```python
from build123d import *

# Parameters (mm, degrees)
ESQUISSE1_R                  = 70
BOSS_EXTRU_1_DEPTH           = 10
CHANFREIN1_SIZE              = 2.12
CHANFREIN1_SIZE2             = 9.973815832
ESQUISSE2_R                  = 1.25
ENL_V_MAT_EXTRU_1_DEPTH      = 8
BOSS_EXTRU_2_START           = 3
ESQUISSE3_R                  = 2.5
ESQUISSE3_R_2                = 1.25
BOSS_EXTRU_2_DEPTH           = 3
R_P_TITION_CIRCULAIRE1_COUNT = 3
ENL_V_MAT_EXTRU_2_REACH      = 101.499
ESQUISSE5_R                  = 1.25
ENL_V_MAT_EXTRU_3_DEPTH      = 8
ENL_V_MAT_EXTRU_4_REACH      = 101.499
ESQUISSE6_R                  = 1.25
BOSS_EXTRU_3_DEPTH           = 5


with BuildPart() as part:
    # Esquisse1 → Boss.-Extru.1 (new body)
    with BuildSketch(Plane.XY):
        Circle(ESQUISSE1_R)
        Polygon((60.258047595, 0), (30.129023798, 52.185), (-30.129023798, 52.185), (-60.258047595, 0), (-30.129023798, -52.185), (30.129023798, -52.185), align=None, mode=Mode.SUBTRACT)
    extrude(amount=BOSS_EXTRU_1_DEPTH)

    # Chanfrein1
    chanfrein1_edges = [part.edges().sort_by_distance(p)[0] for p in [
        (45.193535696, -26.0925, 10),
        (45.193535696, 26.0925, 10),
        (0, 52.185, 10),
        (-45.193535696, 26.0925, 10),
        (-45.193535696, -26.0925, 10),
        (0, -52.185, 10),
    ]]
    chanfrein1_side = [part.faces().sort_by_distance(p)[0] for p in [
        (-68.020101013, 0, 10),
    ]]
    chamfer(chanfrein1_edges, length=CHANFREIN1_SIZE, length2=CHANFREIN1_SIZE2, reference=chanfrein1_side[0])

    # Esquisse2 → Enlèv. mat.-Extru.1 (cut)
    with BuildSketch(Plane(origin=(-43.235330862, -24.961929912, -10.611643989), x_dir=(0.1800568059919566, 0.10395584540888045, -0.9781476007338055), z_dir=(0.8471006708862736, 0.48907380036690296, 0.20791169081776076))):
        with Locations(Location((-16.540417403, 15, 0), (0, 0, 90))):
            Circle(ESQUISSE2_R)
        with Locations(Location((-16.540417403, -15, 0), (0, 0, 90))):
            Circle(ESQUISSE2_R)
    enl_v_mat_extru_1 = extrude(amount=-ENL_V_MAT_EXTRU_1_DEPTH, mode=Mode.SUBTRACT)

    # Esquisse3 → Boss.-Extru.2 (add)
    # profile 1 of 2: a face of its own
    with BuildSketch(Plane(origin=(-43.235330862, -24.961929912, -10.611643989), x_dir=(0.1800568059919566, 0.10395584540888045, -0.9781476007338055), z_dir=(0.8471006708862736, 0.48907380036690296, 0.20791169081776076)).offset(BOSS_EXTRU_2_START)):
        with Locations(Location((-16.540417403, -15, 0), (0, 0, 90))):
            Circle(ESQUISSE3_R)
        with Locations(Location((-16.540417403, -15, 0), (0, 0, 90))):
            Circle(ESQUISSE3_R_2, mode=Mode.SUBTRACT)
    # profile 2 of 2: a face of its own
    with BuildSketch(Plane(origin=(-43.235330862, -24.961929912, -10.611643989), x_dir=(0.1800568059919566, 0.10395584540888045, -0.9781476007338055), z_dir=(0.8471006708862736, 0.48907380036690296, 0.20791169081776076)).offset(BOSS_EXTRU_2_START)):
        with Locations(Location((-16.540417403, 15, 0), (0, 0, 90))):
            Circle(ESQUISSE3_R)
        with Locations(Location((-16.540417403, 15, 0), (0, 0, 90))):
            Circle(ESQUISSE3_R_2, mode=Mode.SUBTRACT)
    boss_extru_2 = extrude(amount=-BOSS_EXTRU_2_DEPTH)

    # Répétition circulaire1: Enlèv. mat.-Extru.1, Boss.-Extru.2 ×3 about axis
    r_p_tition_circulaire1_axis = Axis((0, 0, 0), (0, 0, 1))
    add([enl_v_mat_extru_1.rotate(r_p_tition_circulaire1_axis, i * 360 / R_P_TITION_CIRCULAIRE1_COUNT) for i in range(1, R_P_TITION_CIRCULAIRE1_COUNT)], mode=Mode.SUBTRACT)
    add([boss_extru_2.rotate(r_p_tition_circulaire1_axis, i * 360 / R_P_TITION_CIRCULAIRE1_COUNT) for i in range(1, R_P_TITION_CIRCULAIRE1_COUNT)])

    # Esquisse4 → Enlèv. mat.-Extru.2 (cut, up to next)
    with BuildSketch(Plane(origin=(0, 0, 0), x_dir=(-1, 0, 0), z_dir=(0, 0, -1)), mode=Mode.PRIVATE) as enl_v_mat_extru_2_sk1:
        with BuildLine():
            Line((30.512292605, 63), (-30.512292605, 63))
            ThreePointArc((-30.512292605, 63), (0, 70), (30.512292605, 63))
        make_face()
    enl_v_mat_extru_2_tool1 = extrude(enl_v_mat_extru_2_sk1.sketch, amount=-ENL_V_MAT_EXTRU_2_REACH, mode=Mode.PRIVATE) & part.part
    add(enl_v_mat_extru_2_tool1.solids().sort_by_distance((0, 65.812358, 0))[0], mode=Mode.SUBTRACT)

    # Esquisse5 → Enlèv. mat.-Extru.3 (cut)
    with BuildSketch(Plane(origin=(0, 63, 0), x_dir=(1, 0, 0), z_dir=(0, 1, 0))):
        with Locations(Location((-20, -5, 0), (0, 0, 270))):
            Circle(ESQUISSE5_R)
        with Locations(Location((20, -5, 0), (0, 0, 270))):
            Circle(ESQUISSE5_R)
    extrude(amount=-ENL_V_MAT_EXTRU_3_DEPTH, mode=Mode.SUBTRACT)

    # Esquisse6 → Enlèv. mat.-Extru.4 (cut, up to next)
    with BuildSketch(Plane(origin=(0, 0, 0), x_dir=(-1, 0, 0), z_dir=(0, 0, -1)), mode=Mode.PRIVATE) as enl_v_mat_extru_4_sk1:
        with Locations((48.823972226, 37.179434383)):
            Circle(ESQUISSE6_R)
    enl_v_mat_extru_4_tool1 = extrude(enl_v_mat_extru_4_sk1.sketch, amount=-ENL_V_MAT_EXTRU_4_REACH, mode=Mode.PRIVATE) & part.part
    # Esquisse6 → Enlèv. mat.-Extru.4 (cut, up to next)
    with BuildSketch(Plane(origin=(0, 0, 0), x_dir=(-1, 0, 0), z_dir=(0, 0, -1)), mode=Mode.PRIVATE) as enl_v_mat_extru_4_sk2:
        with Locations((-48.823972226, 37.179434383)):
            Circle(ESQUISSE6_R)
    enl_v_mat_extru_4_tool2 = extrude(enl_v_mat_extru_4_sk2.sketch, amount=-ENL_V_MAT_EXTRU_4_REACH, mode=Mode.PRIVATE) & part.part
    add(enl_v_mat_extru_4_tool1.solids().sort_by_distance((-48.823972, 37.179434, 0))[0], mode=Mode.SUBTRACT)
    add(enl_v_mat_extru_4_tool2.solids().sort_by_distance((48.823972, 37.179434, 0))[0], mode=Mode.SUBTRACT)

    # Esquisse7 → Boss.-Extru.3 (add)
    with BuildSketch(Plane(origin=(0, -52.185, 0), x_dir=(1, 0, 0), z_dir=(0, 1, 0))):
        with BuildLine():
            Line((2, -0.026184168), (4, -0.026184168))
            ThreePointArc((4, -0.026184168), (0, 3.973815832), (-4, -0.026184168))
            Line((-4, -0.026184168), (-2, -0.026184168))
            ThreePointArc((-2, -0.026184168), (0, 1.973815832), (2, -0.026184168))
        make_face()
    extrude(amount=-BOSS_EXTRU_3_DEPTH)


solid = part.part
```
Design review of the part built by this model. Coordinates are the model's own, in mm. A direction names the side the tool comes from. Give positions to 0.01 mm unless a question says otherwise; leave off trailing zeros. Write each loop counter-clockwise with the first axis right and the second up, starting at its lowest first coordinate (ties: lowest second). Pieces come first, ordered by that corner, then holes. Notation, with made-up numbers: (-20, 61.25) - (16, 61.25) arc R14 cw to (16, 68.25) - close; hole circle Ø7 at (84, 12.25). An arc over 180 degrees is marked (long way). Return JSON: item names as keys, results as strings. Group by question number.
(1) To check wall thickness, follow probe 1 along X at (y, z) = (58.25, 5); probe 2 along Z at (x, y) = (63.5, 19.5); probe 3 along Y at (x, z) = (-52.5, 7.5). State the ranges of each line that lie inside material, in increasing order.
(2) Machinability: for faces 3 (the flat face through (46.32, 26.23, 4.94)), 4 (the cylindrical face through (17.385, 52.031, 6.618)), which of the approach directions +Z, -Z, +X, -X, +Y, -Y give a long, thin tool a straight path to every point of the face, cutting with its end or side? Answer none if there is none.
(3) Insertion check: pin 1 (3 mm diameter, centred on x = -12, z = 8.5, fed in from -Y); pin 2 (8 mm diameter, centred on x = -34.5, z = 0, fed in from -Y); pin 3 (5 mm diameter, centred on y = 42, z = -1.5, fed in from +X); pin 4 (1.5 mm diameter, centred on x = 48.82, y = 37.18, fed in from +Z). Each pin has a flat end and moves straight along its axis. Give the tip position at first contact, or say it passes through.
(4) We need section A-A, the plane x = 0. Give the boundary of the cut face in (y, z) (3 decimals).
(5) Mouldability with a two-part tool opening along X and no side actions: class faces 1 (the cylindrical face through (-12.69, 51.68, 4.95)), 2 (the cylindrical face through (-2.64, -69.95, 4.93)) as +X half, -X half, draft (parallel to the pull), parting line (faces both ways), or undercut.
Reported:
{
 "1": {"probe 1": "x = -38.82 to -21.25, -18.75 to -16.16, -13.84 to 13.84, 16.16 to 18.75, 21.25 to 38.82", "probe 2": "z = 0 to 10", "probe 3": "y = -46.3 to -16.61, -14.99 to -10.56, 16.61 to 46.3"},
 "2": {"face 3": "+Z", "face 4": "none"},
 "3": {"pin 1": "stops at y = -69.21", "pin 2": "stops at y = -63.01", "pin 3": "stops at x = 57.45", "pin 4": "passes through"},
 "4": {"outline": "(-70, 0) - (-52.185, 0) - (-52.185, 0.026) - (-54.305, 10) - (-70, 10) - close; (-57.185, -3.974) - (-52.185, -3.974) - (-52.185, -1.974) - (-57.185, -1.974) - close; (52.185, 0) - (63, 0) - (63, 10) - (54.305, 10) - (52.185, 0.026) - close"},
 "5": {"face 1": "undercut", "face 2": "parting line"}
}
